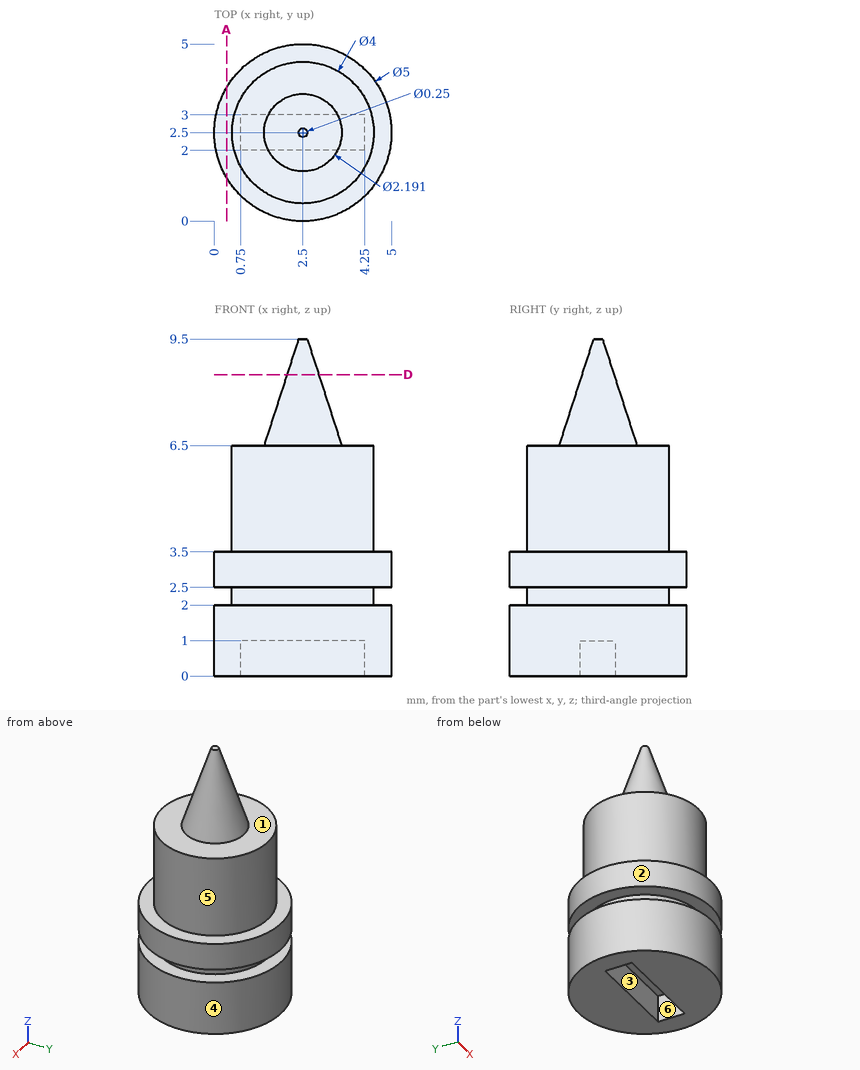
Here's the drawing with two shaded views (mm, measured from the low corner). I have some questions. A direction names the side the tool comes from. Round coordinates to 2 decimals unless told otherwise and drop trailing zeros. Order: outer loops, then holes, each group sorted by start corner. A loop starts at its lowest first (then second) coordinate and runs counter-clockwise, first axis right, second up. Notation, with made-up numbers: (-1.75, 3.5) -> (25.25, 3.5) arc R26 cw to (25.25, 22.5) -> close; hole circle Ø3 at (-23.75, 1). An arc over 180 degrees is marked (long way). Use a Markdown table: item, result. Add a question column.
(1) For pin 1 Ø3 at (x, y) = (4.5, 4.5) entering from +Z; pin 2 Ø1 at (x, z) = (2, 8) entering from +Y; pin 3 Ø0.8 at (x, y) = (1.5, 2.5) entering from -Z, each with a flat end and sliding along its axis, tell me the tip position at first contact or that it passes through.
(2) Suppose I cut it at D-D, the plane z = 8.5. Please give me the cut outline in (x, y), and give its area (3 significant figures).
(3) Suppose I cut it at A-A, the plane x = 0.35. Please give me the cut outline in (y, z).
(4) For the marked faces 4, 5 and 6, which set-ups out of +Z, -Z, +X, -X, +Y, -Y let a thin tool reach every point of the face, with its end or its side?
(5) If we mould it in two halves opening along Y, with no side actions, what happens to the marked faces 1, 2 and 3? For each: released by +Y, released by -Y, zero draft, split by the parting line, or undercut.
(6) I need wall thicknesses on line 1 along Z through (x, y) = (3.25, 0.4); line 2 along Y through (x, z) = (4, 0.5); line 3 along Z through (x, y) = (3.1, 1.4). Which ranges of each line are inside material? Lowest first, please.
Verdict:
| question | item | result |
|---|---|---|
| 1 | pin 1 | z = 6.5 |
| 1 | pin 2 | y = 3.21 |
| 1 | pin 3 | z = 1 |
| 2 | outline | circle Ø0.9 at (2.5, 2.5) |
| 2 | area | 0.632 mm2 |
| 3 | outline | (1.22, 0) -> (3.78, 0) -> (3.78, 2) -> (1.22, 2) -> close; (1.22, 2.5) -> (3.78, 2.5) -> (3.78, 3.5) -> (1.22, 3.5) -> close |
| 4 | face 4 | +Z, -Z |
| 4 | face 5 | +Z |
| 4 | face 6 | -Z |
| 5 | face 1 | zero draft |
| 5 | face 2 | split by the parting line |
| 5 | face 3 | undercut |
| 6 | line 1 | 0 to 2, 2.5 to 3.5 |
| 6 | line 2 | 0.5 to 2, 3 to 4.5 |
| 6 | line 3 | 0 to 6.5 |
